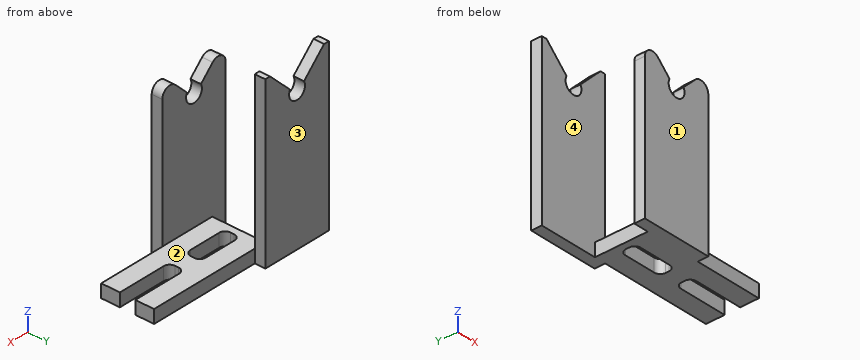
```python
from build123d import *

# Parameters (mm, degrees)
F0_W           = 44.45
F0_H           = 4.7625
F1_DEPTH       = 19.05
F2_W           = 15.875
F2_H           = 5.588
F3_DEPTH       = 4.7635
F4_R           = 2.159
F5_R           = 3.175
F6_DEPTH       = 3.81
F7_W           = 34.26374
F7_H           = 5.588
F8_DEPTH       = 25.4
F10_DEPTH      = 3.811
F10_DEPTH_BACK = 19.051
F11_W          = 25.4
F11_H          = 61.851404
F11_R          = 3.175
F12_DEPTH      = 3.81
F14_DEPTH      = 5.08
F15_R          = 3.048


with BuildPart() as f1:
    # F0 (on Front) → F1 (new body)
    with BuildSketch(Plane.XZ):
        with Locations((-22.225, -83.34375)):
            Rectangle(F0_W, F0_H)
    extrude(amount=F1_DEPTH)

    # F2 (on face) → F3 (cut, through all)
    with BuildSketch(Plane.XY.offset(-80.9625)):
        with Locations((-33.9725, -9.525)):
            Rectangle(F2_W, F2_H)
        with Locations((-11.7475, -9.525)):
            Rectangle(F2_W, F2_H)
    extrude(amount=-F3_DEPTH, mode=Mode.SUBTRACT)

    # F4
    f4_edges = [f1.edges().sort_by_distance(p)[0] for p in [
        (-3.81, -6.731, -83.34375),
        (-26.035, -6.731, -83.34375),
        (-3.81, -12.319, -83.34375),
        (-26.035, -12.319, -83.34375),
        (-19.685, -6.731, -83.34375),
        (-41.91, -6.731, -83.34375),
        (-19.685, -12.319, -83.34375),
        (-41.91, -12.319, -83.34375),
    ]]
    fillet(f4_edges, radius=F4_R)

    # F5 (on Front) → F6 (join)
    with BuildSketch(Plane.XZ):
        Polygon((-65.7225, -85.725), (-44.45, -85.725), (-40.3225, -85.725), (-40.3225, -25.4), (-65.7225, -25.4), align=None)
        with Locations((-53.0225, -34.925)):
            Circle(F5_R, mode=Mode.SUBTRACT)
    extrude(amount=-F6_DEPTH)

    # F7 (on face) → F8 (cut)
    with BuildSketch(Plane(origin=(0, 0, -85.725), x_dir=(1, 0, 0), z_dir=(0, 0, -1))):
        with Locations((6.945667, 9.525)):
            Rectangle(F7_W, F7_H)
    extrude(amount=-F8_DEPTH, mode=Mode.SUBTRACT)

    # F9 (on Front) → F10 (cut, two sides)
    with BuildSketch(Plane.XZ) as f10_sk:
        Polygon((-68.922343, -20.311116), (-53.0225, -36.210959), (-37.122657, -20.311116), align=None)
    extrude(amount=-F10_DEPTH, mode=Mode.SUBTRACT)
    extrude(f10_sk.sketch, amount=-F10_DEPTH_BACK, mode=Mode.SUBTRACT)

    # F11 (on face) → F12 (join)
    with BuildSketch(Plane.XZ.offset(19.05)):
        with Locations((-37.1475, -54.799298)):
            Rectangle(F11_W, F11_H)
        with Locations((-37.1475, -38.1)):
            Circle(F11_R, mode=Mode.SUBTRACT)
    extrude(amount=F12_DEPTH)

    # F13 (on face) → F14 (cut)
    with BuildSketch(Plane.XZ.offset(22.86)):
        Polygon((-55.090682, -21.442777), (-39.9415, -36.591959), (-34.3535, -36.591959), (-19.204318, -21.442777), align=None)
    extrude(amount=-F14_DEPTH, mode=Mode.SUBTRACT)

    # F15
    f15_edges = [f1.edges().sort_by_distance(p)[0] for p in [
        (-49.8475, -20.955, -26.685959),
        (-24.4475, -20.955, -26.685959),
    ]]
    fillet(f15_edges, radius=F15_R)


solid = f1.part
```
Geometry check sheet. Reference: the model listing, model coordinates, mm. Face numbers are marked on the shaded views. Coordinates: 2 decimals unless noted, no trailing zeros. Write each loop counter-clockwise with the first axis right and the second up, starting at its lowest first coordinate (ties: lowest second). Pieces come first, ordered by that corner, then holes. Notation, with made-up numbers: M 27.5,65 L 86.5,65 A17 ccw 86.5,75 Z; hole C -3.5,43 d10. An arc over 180 degrees is marked long. One line per item, written item: value. Start each with the question number.
(1) Depth check by flat-ended pin: pin 1 (4 mm diameter, centred on y = -14, z = -84, fed in from -X); pin 2 (12 mm diameter, centred on y = -11, z = -50.5, fed in from +X); pin 3 (0.6 mm diameter, centred on y = -9.5, z = -83, fed in from +X) (3 decimals); pin 4 (2.5 mm diameter, centred on x = -5, z = -84, fed in from -Y). Enter the tip coordinate at first touch or a pass-through.
(2) Scan lines: line 1 along Y through (x, z) = (-45, -57); line 2 along X through (y, z) = (-20.8, -38.1); line 3 along Z through (x, y) = (-12, -15) (1 decimal). Record each from-to range of solid material in increasing order. Write a range as [from, to].
(3) Sectioned sample at B-B, the plane z = -52.5. Enter the section's corners in (x, y), and give its area (3 significant figures).
(4) Release check for a two-part mould opening along Y. For the marked faces 1, 2, 3 and 4 record: released by +Y, released by -Y, zero draft, split by the parting line, or undercut.
(5) Sectioned sample at C-C, the plane z = -40. Enter the section's corners in (x, y).
Filled sheet:
1. pin 1: x = -44.45
1. pin 2: through
1. pin 3: x = -19.685
1. pin 4: y = -19.05
2. line 1: [-22.86, -19.05], [0, 3.81]
2. line 2: [-49.85, -40.32], [-33.97, -24.45]
2. line 3: [-85.7, -81]
3. outline: M -65.72,0 L -40.32,0 L -40.32,3.81 L -65.72,3.81 Z; M -49.85,-22.86 L -24.45,-22.86 L -24.45,-19.05 L -49.85,-19.05 Z
3. area: 194 mm²
4. face 1: released by -Y
4. face 2: undercut
4. face 3: released by +Y
4. face 4: undercut
5. outline: M -65.72,0 L -40.32,0 L -40.32,3.81 L -65.72,3.81 Z; M -49.85,-22.86 L -39.69,-22.86 L -39.69,-19.05 L -49.85,-19.05 Z; M -34.6,-22.86 L -24.45,-22.86 L -24.45,-19.05 L -34.6,-19.05 Z
